from build123d import *
from build123d.topology import SkipClean

# Parameters (mm, degrees)
BOSS_EXTRUDE1_DEPTH      = 4.7625
BOSS_EXTRUDE1_DEPTH_BACK = 4.7625
SKETCH1_R                = 11.5062
CUT_EXTRUDE1_START       = 3.175
CUT_EXTRUDE1_DEPTH       = 1.5875
CUT_EXTRUDE2_START       = -4.7625
CUT_EXTRUDE2_DEPTH       = 1.5875
FILLET1_R                = 1.5875


with BuildPart() as part:
    # Sketch1 → Boss-Extrude1 (new, two sides: drawn at the far end of the back side and taken through both)
    # profile 1 of 2: a face of its own
    with BuildSketch(Plane.XY.offset(-BOSS_EXTRUDE1_DEPTH_BACK)):
        with BuildLine():
            ThreePointArc((-12.585193267, -7.559797873), (-10.89585042, -11.492870345), (-10.31875, -15.734319794))
            Line((-10.31875, -15.734319794), (-10.31875, -68.439319794))
            Line((-10.31875, -68.439319794), (10.31875, -68.439319794))
            Line((10.31875, -68.439319794), (10.31875, -22.596549828))
            ThreePointArc((10.31875, -22.596549828), (11.166228871, -21.192083745), (12.80382084, -21.287151937))
            Line((12.80382084, -21.287151937), (50.720494758, -47.278411809))
            Line((50.720494758, -47.278411809), (62.388915679, -30.256239225))
            Line((62.388915679, -30.256239225), (18.812153865, -0.385081668))
            ThreePointArc((18.812153865, -0.385081668), (15.640023815, 2.489031981), (13.351109218, 6.106186705))
            ThreePointArc((13.351109218, 6.106186705), (6.843715397, -12.988502339), (-12.585193267, -7.559797873))
        make_face()
        with BuildLine():
            ThreePointArc((5.55625, -58.120569794), (0, -63.676819794), (-5.55625, -58.120569794))
            Line((-5.55625, -58.120569794), (-5.55625, -27.958069794))
            ThreePointArc((-5.55625, -27.958069794), (0, -22.401819794), (5.55625, -27.958069794))
            Line((5.55625, -27.958069794), (5.55625, -58.120569794))
        make_face(mode=Mode.SUBTRACT)
        with BuildLine():
            ThreePointArc((51.185116867, -28.350222438), (52.626511545, -36.074612997), (44.902120986, -37.516007675))
            Line((44.902120986, -37.516007675), (20.023561057, -20.462161714))
            ThreePointArc((20.023561057, -20.462161714), (18.582166378, -12.737771155), (26.306556937, -11.296376477))
            Line((26.306556937, -11.296376477), (51.185116867, -28.350222438))
        make_face(mode=Mode.SUBTRACT)
    # profile 2 of 2: a face of its own
    with BuildSketch(Plane.XY.offset(-BOSS_EXTRUDE1_DEPTH_BACK)):
        with BuildLine():
            ThreePointArc((13.351109218, 6.106186705), (-6.843715397, 12.988502339), (-12.585193267, -7.559797873))
            ThreePointArc((-12.585193267, -7.559797873), (6.843715397, -12.988502339), (13.351109218, 6.106186705))
        make_face()
        Circle(SKETCH1_R, mode=Mode.SUBTRACT)
    extrude(amount=BOSS_EXTRUDE1_DEPTH + BOSS_EXTRUDE1_DEPTH_BACK)

    # Sketch1<8> → Cut-Extrude1 (cut)
    with SkipClean():  # the faces are left unmerged after this step: merging them gives an invalid solid
        with BuildSketch(Plane.XY.offset(CUT_EXTRUDE1_START)):
            with BuildLine():
                ThreePointArc((-12.585193267, -7.559797873), (-10.89585042, -11.492870345), (-10.31875, -15.734319794))
                Line((-10.31875, -15.734319794), (-10.31875, -68.439319794))
                Line((-10.31875, -68.439319794), (10.31875, -68.439319794))
                Line((10.31875, -68.439319794), (10.31875, -22.596549828))
                ThreePointArc((10.31875, -22.596549828), (11.166228871, -21.192083745), (12.80382084, -21.287151937))
                Line((12.80382084, -21.287151937), (50.720494758, -47.278411809))
                Line((50.720494758, -47.278411809), (62.388915679, -30.256239225))
                Line((62.388915679, -30.256239225), (18.812153865, -0.385081668))
                ThreePointArc((18.812153865, -0.385081668), (15.640023815, 2.489031981), (13.351109218, 6.106186705))
                ThreePointArc((13.351109218, 6.106186705), (6.843715397, -12.988502339), (-12.585193267, -7.559797873))
            make_face()
            with BuildLine():
                ThreePointArc((5.55625, -58.120569794), (0, -63.676819794), (-5.55625, -58.120569794))
                Line((-5.55625, -58.120569794), (-5.55625, -27.958069794))
                ThreePointArc((-5.55625, -27.958069794), (0, -22.401819794), (5.55625, -27.958069794))
                Line((5.55625, -27.958069794), (5.55625, -58.120569794))
            make_face(mode=Mode.SUBTRACT)
            with BuildLine():
                ThreePointArc((51.185116867, -28.350222438), (52.626511545, -36.074612997), (44.902120986, -37.516007675))
                Line((44.902120986, -37.516007675), (20.023561057, -20.462161714))
                ThreePointArc((20.023561057, -20.462161714), (18.582166378, -12.737771155), (26.306556937, -11.296376477))
                Line((26.306556937, -11.296376477), (51.185116867, -28.350222438))
            make_face(mode=Mode.SUBTRACT)
        extrude(amount=CUT_EXTRUDE1_DEPTH, mode=Mode.SUBTRACT)

    # Sketch1<9> → Cut-Extrude2 (cut)
    with SkipClean():  # the faces are left unmerged after this step: merging them gives an invalid solid
        with BuildSketch(Plane.XY.offset(CUT_EXTRUDE2_START)):
            with BuildLine():
                ThreePointArc((-12.585193267, -7.559797873), (6.843715397, -12.988502339), (13.351109218, 6.106186705))
                ThreePointArc((13.351109218, 6.106186705), (15.640023815, 2.489031981), (18.812153865, -0.385081668))
                Line((18.812153865, -0.385081668), (62.388915679, -30.256239225))
                Line((62.388915679, -30.256239225), (50.720494758, -47.278411809))
                Line((50.720494758, -47.278411809), (12.80382084, -21.287151937))
                ThreePointArc((12.80382084, -21.287151937), (11.166228871, -21.192083745), (10.31875, -22.596549828))
                Line((10.31875, -22.596549828), (10.31875, -68.439319794))
                Line((10.31875, -68.439319794), (-10.31875, -68.439319794))
                Line((-10.31875, -68.439319794), (-10.31875, -15.734319794))
                ThreePointArc((-10.31875, -15.734319794), (-10.89585042, -11.492870345), (-12.585193267, -7.559797873))
            make_face()
            with BuildLine():
                ThreePointArc((26.306556937, -11.296376477), (18.582166378, -12.737771155), (20.023561057, -20.462161714))
                Line((20.023561057, -20.462161714), (44.902120986, -37.516007675))
                ThreePointArc((44.902120986, -37.516007675), (52.626511545, -36.074612997), (51.185116867, -28.350222438))
                Line((51.185116867, -28.350222438), (26.306556937, -11.296376477))
            make_face(mode=Mode.SUBTRACT)
            with BuildLine():
                ThreePointArc((5.55625, -27.958069794), (0, -22.401819794), (-5.55625, -27.958069794))
                Line((-5.55625, -27.958069794), (-5.55625, -58.120569794))
                ThreePointArc((-5.55625, -58.120569794), (0, -63.676819794), (5.55625, -58.120569794))
                Line((5.55625, -58.120569794), (5.55625, -27.958069794))
            make_face(mode=Mode.SUBTRACT)
        extrude(amount=CUT_EXTRUDE2_DEPTH, mode=Mode.SUBTRACT)

    # Fillet1
    fillet1_edges = [part.edges().sort_by_distance(p)[0] for p in [
        (-10.31875, -68.439319794, 0),
        (10.31875, -68.439319794, 0),
        (50.720494758, -47.278411809, 0),
        (62.388915679, -30.256239225, 0),
    ]]
    fillet(fillet1_edges, radius=FILLET1_R)


solid = part.part
Could you check a few things on this model? Use its own coordinates, in mm. A direction names the side the tool comes from. Give positions to 0.01 mm unless a question says otherwise; leave off trailing zeros. Order: outer loops, then holes, each group sorted by start corner. A loop starts at its lowest first (then second) coordinate and runs counter-clockwise, first axis right, second up. Notation, with made-up numbers: (-7, 20) -> (22, 20) arc R14 ccw to (22, 25) -> close; hole circle Ø9 at (-18.5, 84.25). An arc over 180 degrees is marked (long way). Return JSON: item names as keys, results as strings.
1. Thinking about a two-plate mould opening in X: for faces 1 (the flat face through (-10.319, -41, 0)), 2 (the flat face through (0, -68.439, 0)), 3 (the cylindrical face through (0.122, -63.675, -0.044)), which applies, pulls with the +X half, pulls with the -X half, needs draft (parallel to the pull), parting line crosses it, or undercut?
Answer list:
{"face 1": "pulls with the -X half", "face 2": "needs draft", "face 3": "undercut"}
2. Imagine slicing it at D-D on z = 1.5. Give the number of separate pieces and of enclosed holes in the cut face, then the cut area to 3 significant figures.
Answer list:
{"separate pieces": "1", "enclosed holes": "3", "area": "1,650 mm2"}
3. Imagine slicing it at A-A on x = 0. List the corners of the cut face in (y, z) for me (1 decimal), then the cut area to 3 significant figures.
Answer list:
{"outline": "(-68.4, -3.2) -> (-63.7, -3.2) -> (-63.7, 3.2) -> (-68.4, 3.2) -> close; (-22.4, -3.2) -> (-14.7, -3.2) -> (-14.7, -4.8) -> (-11.5, -4.8) -> (-11.5, 4.8) -> (-14.7, 4.8) -> (-14.7, 3.2) -> (-22.4, 3.2) -> close; (11.5, -4.8) -> (14.7, -4.8) -> (14.7, 4.8) -> (11.5, 4.8) -> close", "area": "140 mm2"}
4. Imagine slicing it at B-B on y = -53. List the corners of the cut face in (x, z) for me (3 decimals), then the cut area to 3 significant figures.
Answer list:
{"outline": "(-10.319, -3.175) -> (-5.556, -3.175) -> (-5.556, 3.175) -> (-10.319, 3.175) -> close; (5.556, -3.175) -> (10.319, -3.175) -> (10.319, 3.175) -> (5.556, 3.175) -> close", "area": "60.5 mm2"}
5. Imagine slicing it at C-C on y = -27. List the corners of the cut face in (x, z) for me (3 decimals).
Answer list:
{"outline": "(-10.319, -3.175) -> (-5.473, -3.175) -> (-5.473, 3.175) -> (-10.319, 3.175) -> close; (5.473, -3.175) -> (10.319, -3.175) -> (10.319, 3.175) -> (5.473, 3.175) -> close; (21.138, -3.175) -> (29.561, -3.175) -> (29.561, 3.175) -> (21.138, 3.175) -> close; (49.215, -3.175) -> (57.639, -3.175) -> (57.639, 3.175) -> (49.215, 3.175) -> close"}
6. On a 3-axis mill with a long thin cutter (end or side, diameter ignored), from which of +Z, -Z, +X, -X, +Y, -Y can I reach the whole of each face in a straight line? I mean faces 4 (the cylindrical face through (-10.912, -11.435, -0.044)), 5 (the flat face through (10.319, -45, 0)), 6 (the flat face through (5.556, -43, 0)). Say none if no direction works.
Answer list:
{"face 4": "+Z, -Z, -X, -Y", "face 5": "+Z, -Z, -Y", "face 6": "+Z, -Z"}
7. I need wall thicknesses on line 1 (Y direction, x = 0, z = 1.25); line 2 (X direction, y = -51.5, z = -1.75); line 3 (X direction, y = -31, z = -2.25). Which ranges of each line are inside material? Lowest first, please. Write a range as from..to.
Answer list:
{"line 1": "y = -68.44..-63.68, -22.4..-11.51, 11.51..14.68", "line 2": "x = -10.32..-5.56, 5.56..10.32", "line 3": "x = -10.32..-5.56, 5.56..10.32, 26.97..35.4, 53.25..61.73"}
8. For pin 1 Ø5 at (x, z) = (19, -2) entering from -Y; pin 2 Ø3 at (x, z) = (7.5, 2.5) entering from +Y; pin 3 Ø3 at (y, z) = (-45.5, -0.5) entering from -X; pin 4 Ø5 at (x, y) = (15, 5) entering from -Z, each with a flat end and sliding along its axis, tell me the tip position at first contact or that it passes through.
Answer list:
{"pin 1": "stops at y = -27.25", "pin 2": "stops at y = 13.4", "pin 3": "stops at x = -10.32", "pin 4": "stops at z = -4.76"}
